Build history of the part. All positions in model axes, mm. A direction names the side the tool comes from. Round coordinates to 2 decimals unless told otherwise and drop trailing zeros. Loops run counter-clockwise (first coordinate to the right, second up) from the corner with the lowest first, then second, coordinate; pieces in that order, holes last.
from build123d import *

# Parameters (mm, degrees)
F0_W     = 75
F0_H     = 100
F1_DEPTH = 50


with BuildPart() as f1:
    # F0 (on Top) → F1 (new body)
    with BuildSketch(Plane.XY):
        Rectangle(F0_W, F0_H)
    extrude(amount=-F1_DEPTH)

    # F2 (on Right) → F3 (revolve)
    with BuildSketch(Plane.YZ):
        Polygon((0, 0), (0, 188), (-10, 188), (-37.5, 0), align=None)
    revolve(axis=Axis((0, 0, 94), (0, 0, -1)))


solid = f1.part
(1) Pin check, flat tips, straight feed: P1, Ø4, axis at x = 29, y = -38.5, coming from the +Z side; P2, Ø3, axis at x = 9, z = 37.5, coming from the +Y side. Stop position of each tip, or through.
Responses:
P1: stops at z = 0
P2: stops at y = 31.19
(2) Slice it at C-C on z = 105.5. List the corners of the cut face in (x, y).
Responses:
outline: circle Ø44.14 at (0, 0)
(3) Which spindle directions (+Z, -Z, +X, -X, +Y, -Y) get a long thin tool onto all of the face, cutting with end or side? Do faces 1 (the face through (-1, 42, 0)), 2 (the face through (0, 0, 188)), 3 (the face through (-1, -41, 0)). Say none if no direction does.
Responses:
face 1: +Z, +Y
face 2: +Z, +X, -X, +Y, -Y
face 3: +Z, -Y
(4) Slice it at A-A on x = 0. List the corners of the cut face in (y, z).
Responses:
outline: (-50, -50) - (50, -50) - (50, 0) - (37.5, 0) - (10, 188) - (-10, 188) - (-37.5, 0) - (-50, 0) - close
(5) Slice it at B-B on z = 7. List the corners of the cut face in (x, y).
Responses:
outline: circle Ø72.95 at (0, 0)
(6) Probe line 1 (Z direction, x = 27.5, y = -39); line 2 (Y direction, x = 27.5, z = 34.5); line 3 (Y direction, x = 3.5, z = 143). List the from-to ranges inside material, lowest first.
Responses:
line 1: z = -50 to 0
line 2: y = -17.23 to 17.23
line 3: y = -16.21 to 16.21
